Autodesk Inventor part; units mm, degrees
ref_plane "YZ Plane" through (0, 0, 0) normal (1, 0, 0) x (0, 1, 0)
ref_plane "XZ Plane" through (0, 0, 0) normal (0, 1, 0) x (-1, 0, 0)
ref_plane "XY Plane" through (0, 0, 0) normal (0, 0, 1) x (1, 0, 0)
sketch "Sketch1" plane through (0, 0, 0) normal (0, 0, 1) x (1, 0, 0)
  line L0 (-2.5, 25) -> (2.5, 25)
  line L1 (7.5, 20) -> (7.5, -20)
  line L2 (2.5, -25) -> (-2.5, -25)
  line L3 (-7.5, -20) -> (-7.5, 20)
  line L4 (-7.5, 25) -> (7.5, -25) construction
  line L5 (7.5, 25) -> (-7.5, -25) construction
  arc A0 (-2.5, 25) -> (-7.5, 20) centre (-2.5, 20) ccw
  arc A1 (7.5, 20) -> (2.5, 25) centre (2.5, 20) ccw
  arc A2 (2.5, -25) -> (7.5, -20) centre (2.5, -20) ccw
  arc A3 (-7.5, -20) -> (-2.5, -25) centre (-2.5, -20) ccw
  circle A4 centre (0, 20) radius 1
  point P0 (0, 0)
  dimension "d0" = 15
  dimension "d1" = 50
  dimension "d2" = 5
  dimension "d5" = 2
extrude "Extrusion2" add sketch "Sketch1" along normal blind 5
sketch "Sketch3" plane through (0, 0, 5) normal (0, 0, 1) x (1, 0, 0)
  circle A0 centre (0, 20) radius 1
  point P0 (0, 0)
hole "Hole1" at (0, 20, 5) direction (0, 0, -1) diameter 4 end through all countersink diameter 6 countersink angle 90
sketch "Sketch4" plane through (0, 0, 0) normal (1, 0, 0) x (0, 1, 0)
  line L0 (28.9186, 2.2501) -> (-11.8341, 2.2501) construction
  line L1 (20, 0) -> (-20, 0)
  line L2 (-20, 5) -> (20, 5) construction
  line L3 (-2.191, 5) -> (-11.8341, 5) construction
  line L4 (-7.253, 15) -> (-7.253, 5)
  arc A0 (7.747, 30) -> (-7.253, 15) centre (7.747, 15) ccw
  line L5 (7.747, 30) -> (15.747, 30)
  point P0 (0, 0)
  point P1 (8.5422, 2.2501)
  dimension "d24" = 10
  dimension "d25" = 8
sketch "Sketch5" plane through (0, 0, 5) normal (0, 0, 1) x (1, 0, 0)
  line L0 (7.5, 20) -> (7.5, -20)
  line L1 (-7.5, -4.5373) -> (7.5, -4.5373)
  line L2 (7.5, -4.5373) -> (7.5, -9.5373)
  line L3 (7.5, -9.5373) -> (-7.5, -9.5373)
  line L4 (-7.5, -9.5373) -> (-7.5, -4.5373)
  line L5 (-7.5, -4.5373) -> (7.5, -9.5373) construction
  line L6 (7.5, -4.5373) -> (-7.5, -9.5373) construction
  point P0 (0, 0)
  point P1 (0, -7.0373)
  dimension "d17" = 15
  dimension "d18" = 5
sweep "Sweep3" add profiles "Sketch5" path "Sketch4" path curves L4 A0 L5
sketch "Sketch8" plane through (0, 0, 5) normal (0, 0, 1) x (1, 0, 0)
  line L0 (7.5, -9.5373) -> (-7.5, -9.5373)
  line L1 (-7.5, -4.5373) -> (7.5, -4.5373)
  point P0 (0, 0)
sketch "Sketch9" plane through (7.5, -20, 0) normal (1, 0, 0) x (0, 0, -1)
  line L0 (-5, 10.4627) -> (-15.4627, 10.4627)
  line L1 (-5, 10.4627) -> (-15.4627, 10.4627)
  line L2 (-5, 10.4627) -> (-15.4627, 10.4627)
  line L3 (-5, 10.4627) -> (-5, 0)
  line L4 (-5, 10.4627) -> (-5, 0)
  arc A0 (-5, 0) -> (-15.4627, 10.4627) centre (-15.4627, 0) ccw
  point P0 (0, 20)
  dimension "d31" = 10.4627
  dimension "d32" = 10.4627
sweep "Sweep4" add profiles "Sketch9" path "Sketch8" path curves L0
sketch "Sketch10" plane through (-7.5, -20, 0) normal (-1, 0, 0) x (0, 0, 1)
  line L0 (27.2843, 27.747) -> (27.2843, 35.747)
  line L1 (32.2843, 27.747) -> (32.2843, 35.747)
  line L2 (27.2843, 35.747) -> (32.2843, 35.747)
  arc A0 (32.2843, 33.247) -> (27.2843, 33.247) centre (29.7843, 33.247) ccw
  line L3 (27.2843, 33.247) -> (27.2843, 35.747)
  line L4 (32.2843, 35.747) -> (32.2843, 33.247)
  line L5 (27.2843, 35.747) -> (32.2843, 35.747)
  point P0 (0, 20)
  point P1 (29.7843, 35.747)
extrude "Extrusion3" cut sketch "Sketch10" against normal through all
sketch "Sketch11" plane through (-7.5, -4.5373, 5) normal (0, 1, 0) x (1, 0, 0)
  line L0 (0, 0) -> (15, 0)
  point P0 (7.5, 5)
sketch "Sketch12" plane through (-7.5, -20, 0) normal (-1, 0, 0) x (0, 0, 1)
  line L0 (5, 40) -> (5, 15.4627)
  line L1 (5, 15.4627) -> (15, 15.4627)
  line L2 (5, 15.4627) -> (15, 15.4627)
  line L3 (5, 15.4627) -> (5, 25.4627)
  line L4 (5, 15.4627) -> (5, 40)
  arc A0 (5, 25.4627) -> (15, 15.4627) centre (15, 25.4627) ccw
  point P0 (0, 20)
  dimension "d37" = 10
sweep "Sweep5" add profiles "Sketch12" path "Sketch11"
sketch "Sketch15" plane through (-7.5, -20, 0) normal (-1, 0, 0) x (0, 0, 1)
  arc A0 (5, 25.4627) -> (15, 15.4627) centre (15, 25.4627) ccw
  arc A1 (15, 15.4627) -> (27.2843, 27.747) centre (15, 27.747) ccw
  line L0 (15.4627, 10.4627) -> (5, 10.4627)
  arc A2 (0, 15.4627) -> (5, 10.4627) centre (5, 15.4627) ccw
  line L1 (0, 0) -> (0, -5)
  line L2 (0, -5) -> (5, -5)
  line L3 (5, -5) -> (5, 0)
  arc A3 (15.4627, 10.4627) -> (5, 0) centre (15.4627, 0) ccw
  line L4 (0, 0) -> (5, 0)
  line L5 (0, 0) -> (0, 15.4627)
  point P0 (0, 20)
  dimension "d43" = 5
extrude "Extrusion5" cut sketch "Sketch15" against normal through all
fillet "Fillet1" radius 1 33 edges at (7.5, -0.9393, 23.6863) (7.5, 10.497, 27.2843) (7.5, 15.747, 29.7843) (-7.5, 10.497, 32.2843) (-7.5, -4.4748, 27.2219) (-7.5, -9.5373, 10) (7.5, 10.497, 32.2843) (7.5, -4.4748, 27.2219) (7.5, -9.5373, 10) (0, 13.247, 32.2843) (0, 7.747, 32.2843) (0, -9.5373, 15) (0, -9.5373, 5) (7.5, -8.0728, 1.4645) (7.5, 7.7314, 0) (6.0355, 23.5355, 0) (0, 25, 0) (-6.0355, 23.5355, 0) (-7.5, 7.7314, 0) (-7.5, -8.0728, 1.4645) (-7.5, 15.747, 29.7843) (0, -4.5373, 15) (0, 7.747, 27.2843) (-7.5, -0.9393, 23.6863) (-7.5, 10.497, 27.2843) (0, 13.247, 27.2843) (-7.5, -1.6084, 7.9289) (-7.5, 12.7314, 5) (-6.0355, 23.5355, 5) (0, 25, 5) (6.0355, 23.5355, 5) (7.5, 12.7314, 5) (7.5, -1.6084, 7.9289)
sketch "Sketch13" plane through (7.5, -20, 0) normal (1, 0, 0) x (0, 0, -1)
  arc A0 (-5, 0) -> (-15.4627, 10.4627) centre (-15.4627, 0) ccw
  line L0 (0, 0) -> (0, 9.0751)
  line L1 (0, 0) -> (0, 40)
  line L2 (0, -5) -> (0, 0)
  arc A1 (-5, 0) -> (0, 0) centre (-2.5, 0) ccw
  line L3 (0, -5) -> (-5, -5)
  line L4 (0, -5) -> (-5, -5)
  line L5 (-5, 0) -> (-5, -5)
  line L6 (-5, -5) -> (-5, 0)
  point P0 (0, 20)
equation "\"d31\" = d32"
properties part number "single_hook"
Part model, mm, in its own coordinate system. A direction names the side the tool comes from. Give positions to 0.01 mm unless a question says otherwise; leave off trailing zeros. Order: outer loops, then holes, each group sorted by start corner. A loop starts at its lowest first (then second) coordinate and runs counter-clockwise, first axis right, second up. Notation, with made-up numbers: (-16, 47) - (36, 47) arc R23 cw to (36, 81) - close; hole circle Ø10 at (-1.5, 20). An arc over 180 degrees is marked (long way). Use one line per item in the form item = value.
Item 1: Slice it at B-B on y = 9.5. Give the cut face in (x, z).
Solution:
outline = (-7.5, 1) arc R1 ccw to (-6.5, 0) - (6.5, 0) arc R1 ccw to (7.5, 1) - (7.5, 4) arc R1 ccw to (6.5, 5) - (-6.5, 5) arc R1 ccw to (-7.5, 4) - close; (-7.5, 28.28) arc R1 ccw to (-6.5, 27.28) - (6.5, 27.28) arc R1 ccw to (7.5, 28.28) - (7.5, 31.28) arc R1 ccw to (6.5, 32.28) - (-6.5, 32.28) arc R1 ccw to (-7.5, 31.28) - close
Item 2: Two-plate mould, pull along Y, no slides. Class faces 1 (the face through (7.2, 10.46, 27.57)), 2 (the face through (-7.2, -9.25, 9.93)), 3 (the face through (1.2, 21.6, 2)): released by +Y, released by -Y, zero draft, split by the parting line, or undercut.
Solution:
face_1 = zero draft
face_2 = released by -Y
face_3 = undercut
Item 3: Pin check, flat tips, straight feed: pin 1 Ø5 at (y, z) = (11.5, 27.5) entering from -X; pin 2 Ø1.5 at (x, z) = (-2.5, 25.5) entering from +Y; pin 3 Ø6 at (x, z) = (-5, 15) entering from +Y. Stop position of each tip, or through.
Solution:
pin_1 = -7.5
pin_2 = 2.81
pin_3 = -4.08
Item 4: Probe probe 1 along Z at (x, y) = (2, 12); probe 2 along X at (y, z) = (20, 0.95); probe 3 along Y at (x, z) = (0, 2.65). List the from-to ranges inside material, lowest first. Write a range as from..to.
Solution:
probe_1 = 0..5, 27.28..32.28
probe_2 = -7.5..-2, 2..7.5
probe_3 = -8.95..18, 22..25
Item 5: Slice it at A-A on x = 0. Give the cut face in (y, z).
Solution:
outline = (-9.54, 5) arc R5 ccw to (-4.54, 0) - (18, 0) - (18, 4) - (17, 5) - (5.46, 5) arc R10 cw to (-4.54, 15) arc R12.28 cw to (7.75, 27.28) - (13.25, 27.28) arc R2.5 ccw to (13.25, 32.28) - (7.75, 32.28) arc R17.28 ccw to (-9.54, 15) - close; (22, 0) - (24, 0) arc R1 ccw to (25, 1) - (25, 4) arc R1 ccw to (24, 5) - (23, 5) - (22, 4) - close
Item 6: Which spindle directions (+Z, -Z, +X, -X, +Y, -Y) get a long thin tool onto all of the face, cutting with end or side? Do faces 4 (the face through (-0.091, -8.034, 1.426)), 5 (the face through (-7.2, 10.54, 27.57)). Say none if no direction does.
Solution:
face_4 = -Z, +X, -X, -Y
face_5 = -X, +Y
